Verification items for the finished model (mm, model axes). A direction names the side the tool comes from. Coordinates: 2 decimals unless noted, no trailing zeros. Order: outer loops, then holes, each group sorted by start corner. A loop starts at its lowest first (then second) coordinate and runs counter-clockwise, first axis right, second up. Notation, with made-up numbers: M 73.5,32 L 113.5,32 A13 ccw 113.5,36 Z; hole C 51,67.5 d4. An arc over 180 degrees is marked long. Return JSON: item names as keys, results as strings. Group by question number.
Q1. Thickness scan on probe 1 along X at (y, z) = (-9.5, -3); probe 2 along Z at (x, y) = (56, -11); probe 3 along Y at (x, z) = (26, -20.5). Record the ranges inside material, lowest first.
Q2. Mould release check, pull along Y, two halves, no side actions. Record for faces 1 (the face through (-41, 9.525, -20)), 2 (the face through (-49.99, -14, -20)), 3 (the face through (-41, -28.448, -20)): pulls with the +Y half, pulls with the -Y half, needs draft (parallel to the pull), parting line crosses it, or undercut.
Q3. Section check A-A, the plane z = -16.5. Enter the section's corners in (x, y) (3 decimals).
Q4. Section check D-D, the plane z = 0. Enter the section's corners in (x, y).
Q5. Section check C-C, the plane x = 64. Enter the section's corners in (y, z), then the cut area to 3 significant figures.
Q6. Go/stop test with flat-tipped pins: pin 1 Ø5.5 at (y, z) = (-14, 8.5) entering from -X; pin 2 Ø1.5 at (y, z) = (-21, -1) entering from -X; pin 3 Ø19 at (x, z) = (-13, -11) entering from +Y; pin 4 Ø2 at (y, z) = (-5.5, -9.5) entering from -X. Record where each tip stops, or that it passes through.
Q7. Access from +Z, -Z, +X, -X, +Y, -Y to the whole of each face (thin tool, end or side, straight path). Record for faces 4 (the face through (-49.896, 5, -20)), 5 (the face through (-30.846, 5, -20)), 6 (the face through (-30.752, -24, -20)), 7 (the face through (40, -9, 2.441)).
from build123d import *

# Parameters (mm, degrees)
F1_DEPTH = 19.05
F3_DEPTH = 9.525
F4_W     = 19.237377
F4_H     = 19.237377
F5_DEPTH = 28.448


with BuildPart() as f1:
    # F0 (on Front) → F1 (new body)
    with BuildSketch(Plane.XZ):
        Polygon((-24.528947, 34.191047), (-49.928947, 34.191047), (-49.928947, -29.308953), (77.071053, -29.308953), (77.071053, 2.441047), (0.871053, 2.441047), align=None)
    extrude(amount=F1_DEPTH)

    # F2 (on Front) → F3 (join)
    with BuildSketch(Plane.XZ):
        Polygon((-49.896031, -10.243278), (-49.896031, -29.293278), (-30.846031, -29.293278), (-30.846031, -10.055901), align=None)
    extrude(amount=-F3_DEPTH)

    # F4 (on Front) → F5 (join)
    with BuildSketch(Plane.XZ):
        with Locations((-40.371031, -19.674589)):
            Rectangle(F4_W, F4_H)
    extrude(amount=F5_DEPTH)


solid = f1.part
Numbers:
{
 "1": {"probe 1": "x = -49.93 to 77.07", "probe 2": "z = -29.31 to 2.44", "probe 3": "y = -19.05 to 0"},
 "2": {"face 1": "pulls with the +Y half", "face 2": "needs draft", "face 3": "pulls with the -Y half"},
 "3": {"outline": "M -49.99,-28.448 L -30.752,-28.448 L -30.752,-19.05 L 77.071,-19.05 L 77.071,0 L -30.846,0 L -30.846,9.525 L -49.896,9.525 L -49.896,0 L -49.99,0 Z"},
 "4": {"outline": "M -49.93,-19.05 L 77.07,-19.05 L 77.07,0 L -49.93,0 Z"},
 "5": {"outline": "M -19.05,-29.31 L 0,-29.31 L 0,2.44 L -19.05,2.44 Z", "area": "605 mm2"},
 "6": {"pin 1": "stops at x = -49.93", "pin 2": "passes through", "pin 3": "stops at y = 0", "pin 4": "stops at x = -49.99"},
 "7": {"face 4": "+Z, -Z, -X, +Y", "face 5": "+Z, -Z, +X, +Y", "face 6": "+Z, -Z, +X, -Y", "face 7": "+Z, +X, +Y, -Y"}
}
